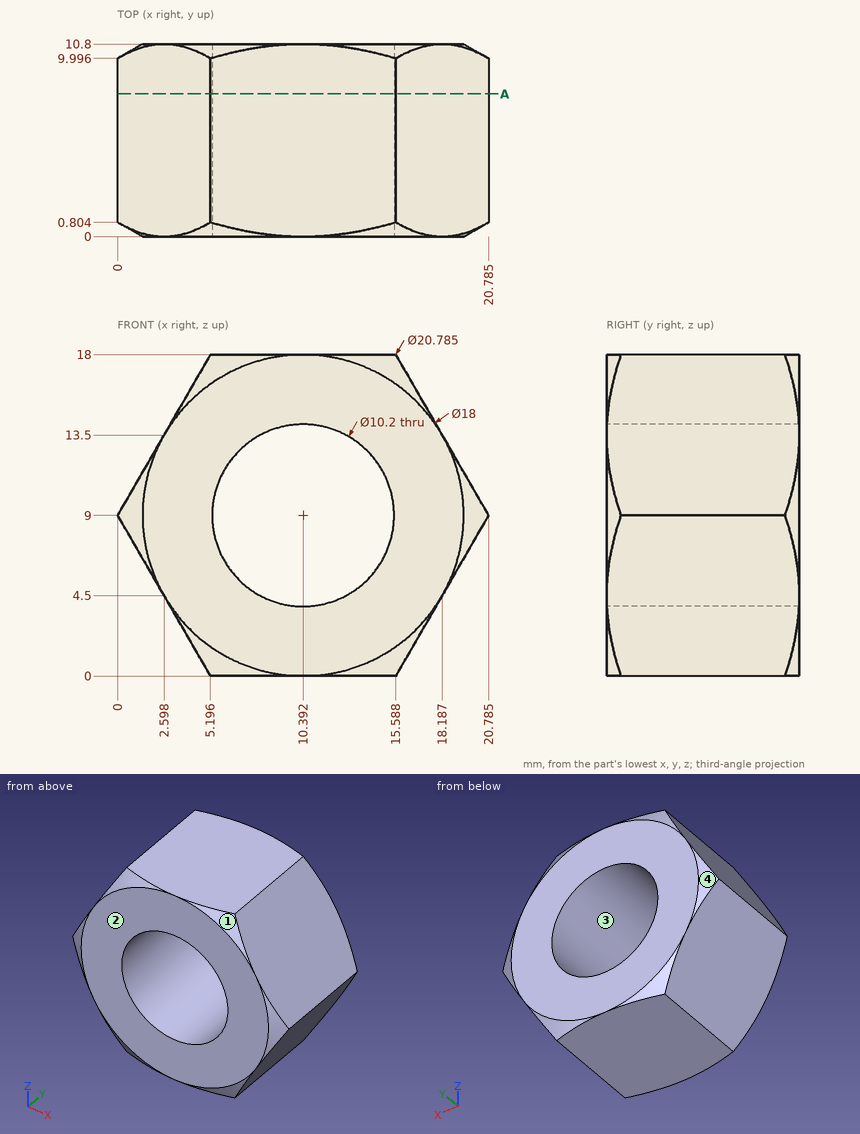
Job drawing, mm, ordinate dimensions from the low corner. One solid piece. Coordinates: 2 decimals unless noted, no trailing zeros. Order: outer loops, then holes, each group sorted by start corner. A loop starts at its lowest first (then second) coordinate and runs counter-clockwise, first axis right, second up. Notation, with made-up numbers: (1, 18) - (6, 18) arc R23 ccw to (6, 28) - close; hole circle Ø9 at (-39.75, -22.5). An arc over 180 degrees is marked (long way). Write each question's results on one line, items separated by ' | '. Start each with the question number.
Item 1: Band-saw the part on A-A on y = 8. Write the cut outline in (x, z) (1 decimal), and give its area (3 significant figures).
Item 2: Mould opens along X. For the marked faces 1, 2, 3 and 4 say: released by +X, released by -X, zero draft, split by the parting line, or undercut.
Item 3: Flat gauge pins, fed straight in: pin 1 (4 mm diameter, centred on y = 6, z = 15, fed in from -X); pin 2 (1.5 mm diameter, centred on y = 7, z = 7, fed in from +X). Where does each tip first touch, or does it go through?
Item 4: Wall check: probe 1 along Z at (x, y) = (6.5, 2) (1 decimal); probe 2 along Z at (x, y) = (9.5, 1.75); probe 3 along X at (y, z) = (6, 10.75) (1 decimal). Give the ranges that are in metal, low to high. Write a range as [from, to].
Numbers:
1) outline: (0, 9) - (5.2, 0) - (15.6, 0) - (20.8, 9) - (15.6, 18) - (5.2, 18) - close; hole circle Ø10.2 at (10.4, 9) | area: 199 mm^2
2) face 1: released by +X | face 2: zero draft | face 3: undercut | face 4: released by -X
3) pin 1: x = 2.31 | pin 2: x = 20.06
4) probe 1: [0, 5.7], [12.3, 18] | probe 2: [0, 3.98], [14.02, 18] | probe 3: [1, 5.6], [15.2, 19.8]
